Read the model definition and answer for the solid it produces. Units are mm, in the model's axes. A direction names the side the tool comes from. Give positions to 0.01 mm unless a question says otherwise; leave off trailing zeros. Order: outer loops, then holes, each group sorted by start corner. A loop starts at its lowest first (then second) coordinate and runs counter-clockwise, first axis right, second up. Notation, with made-up numbers: (84.25, 38.5) - (105.25, 38.5) arc R28 cw to (105.25, 65.5) - close; hole circle Ø1 at (-34, -5.5). An arc over 180 degrees is marked (long way). Use a Markdown table: item, result. Add a question column.
1. Flat-ended cylindrical pins translate along their axes: P1, Ø7, axis at y = 18.5, z = -75.5, coming from the -X side; P2, Ø1.5, axis at y = 10.5, z = -54.5, coming from the -X side; P3, Ø9.5, axis at y = 18, z = -23, coming from the -X side. Find the tip coordinate at first contact, or state that the pin passes through.
2. A cutting plane is placed at D-D on z = -49. Determine the outline of the cut face in (x, y).
3. A cutting plane is placed at B-B on z = -66. Determine the outline of the cut face in (x, y).
4. Consider L1, parallel to Z at x = 57.5, y = 26.25; L2, parallel to X at y = 7.5, z = -28; L3, parallel to X at y = 2, z = -70. Determine where each line is inside the solid, lowest interval first.
5. Which of the six approach directions +Z, -Z, +X, -X, +Y, -Y give full straight-line access (tool end or side, diameter ignored) to faces 4 (the flat face through (52.51, 14, -58)), 5 (the flat face through (43.23, 14.3, -28.4)), 6 (the flat face through (38.274, 14.297, -65.167))?
6. A cutting plane is placed at C-C on x = 31. Determine the outline of the cut face in (y, z).
7. A cutting plane is placed at A-A on z = -35.5. Determine the outline of the cut face in (x, y), and give its area (3 significant figures).
8. For a pull along Z with two mould halves and no side action, classify faces 1 (the flat face through (55, 14, -61.141)), 2 (the flat face through (19.99, 14.3, -71.01)), 3 (the flat face through (47, 14, -25.424)) as released by +Z, released by -Z, zero draft, split by the parting line, or undercut.
```python
from build123d import *

# Parameters (mm, degrees)
BOSS_EXTRUDE1_DEPTH = 29


with BuildPart() as part:
    # Sketch1 → Boss-Extrude1 (new body)
    with BuildSketch(Plane(origin=(0, 0, 0), x_dir=(1, 0, 0), z_dir=(0, 1, 0))):
        Polygon((24.759890606, 17.762425379), (28.759890606, 29.702343473), (29.307835455, 25.423793289), (33.259890606, 25.423793289), (37.259890606, 31.293559553), (39.259890606, 36.702343473), (41.259890606, 31.293559553), (45.259890606, 25.423793289), (49.211945756, 25.423793289), (49.759890606, 29.702343473), (53.759890606, 17.762425379), (57.818331734, 17.762425379), (57.818331734, 26.457588678), (59.259890606, 29.980893658), (58.200604263, 38.06142419), (52.509890606, 38.06142419), (52.509890606, 43.377759071), (48.759890606, 45.399346339), (48.759890606, 53.802982108), (52.509890606, 55.824569376), (52.509890606, 61.140904257), (58.200604263, 61.140904257), (59.259890606, 69.221434789), (57.818331734, 72.744739769), (57.818331734, 81.439903068), (53.759890606, 81.439903068), (49.759890606, 69.499984974), (49.211945756, 73.778535158), (45.259890606, 73.778535158), (41.259890606, 67.908768894), (39.259890606, 62.499984974), (37.259890606, 67.908768894), (33.259890606, 73.778535158), (29.307835455, 73.778535158), (28.759890606, 69.499984974), (24.759890606, 81.439903068), (20.701449477, 81.439903068), (20.701449477, 72.744739769), (19.259890606, 69.221434789), (20.319176948, 61.140904257), (26.009890606, 61.140904257), (26.009890606, 55.824569376), (29.759890606, 53.802982108), (29.759890606, 45.399346339), (26.009890606, 43.377759071), (26.009890606, 38.06142419), (20.319176948, 38.06142419), (19.259890606, 29.980893658), (20.701449477, 26.457588678), (20.701449477, 17.762425379), align=None)
    extrude(amount=BOSS_EXTRUDE1_DEPTH)


solid = part.part
```
Output values:
| question | item | result |
|---|---|---|
| 1 | P1 | x = 20.4 |
| 1 | P2 | x = 27.08 |
| 1 | P3 | x = 20.17 |
| 2 | outline | (29.76, 0) - (48.76, 0) - (48.76, 29) - (29.76, 29) - close |
| 3 | outline | (19.68, 0) - (37.97, 0) - (37.97, 29) - (19.68, 29) - close; (40.55, 0) - (58.84, 0) - (58.84, 29) - (40.55, 29) - close |
| 4 | L1 | -81.44 to -61.14, -38.06 to -17.76 |
| 4 | L2 | 20.07 to 28.19, 28.98 to 35.02, 43.5 to 49.54, 50.33 to 58.45 |
| 4 | L3 | 19.58 to 28.59, 28.82 to 35.83, 42.68 to 49.7, 49.93 to 58.94 |
| 5 | face 4 | +X, +Y, -Y |
| 5 | face 5 | +Z, +Y, -Y |
| 5 | face 6 | -Z, +Y, -Y |
| 6 | outline | (0, -73.78) - (29, -73.78) - (29, -25.42) - (0, -25.42) - close |
| 7 | outline | (19.98, 0) - (38.82, 0) - (38.82, 29) - (19.98, 29) - close; (39.7, 0) - (58.54, 0) - (58.54, 29) - (39.7, 29) - close |
| 7 | area | 1,090 mm² |
| 8 | face 1 | undercut |
| 8 | face 2 | released by -Z |
| 8 | face 3 | released by +Z |
